For this review, take the finished solid that the model builds, in its own axes (mm). Face numbers are marked on the shaded views. A direction names the side the tool comes from. Round coordinates to 2 decimals unless told otherwise and drop trailing zeros. Order: outer loops, then holes, each group sorted by start corner. A loop starts at its lowest first (then second) coordinate and runs counter-clockwise, first axis right, second up. Notation, with made-up numbers: M 72,3 L 116,3 A15 ccw 116,27 Z; hole C -31.5,67.5 d4. An arc over 180 degrees is marked long. Answer as a JSON object with one key per item and string values.
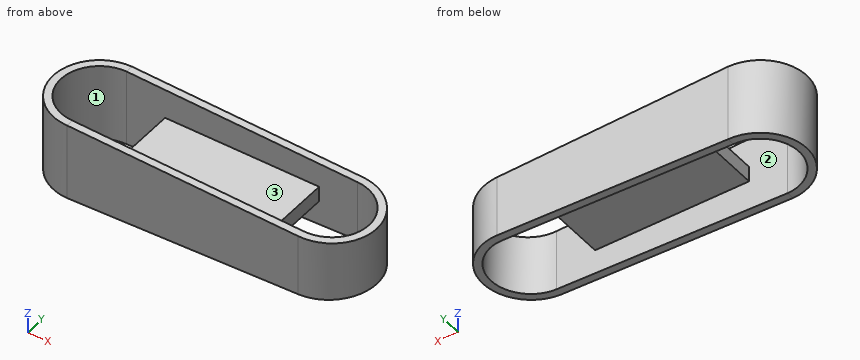
from build123d import *

# Parameters (mm, degrees)
BOSS_EXTRUDE1_DEPTH = 10
SKETCH2_W           = 20
SKETCH2_H           = 2
BOSS_EXTRUDE2_DEPTH = 10
CUT_EXTRUDE1_START  = -12
CUT_EXTRUDE1_DEPTH  = 12


# Read off the part's stored shape, not the designer's step: Cut-Extrude1
with BuildPart() as part:
    # Sketch1 → Boss-Extrude1 (new body)
    with BuildSketch(Plane.XY):
        with BuildLine():
            Line((0, -6), (-30, -6))
            ThreePointArc((-30, -6), (-36, 0), (-30, 6))
            Line((-30, 6), (0, 6))
            ThreePointArc((0, 6), (6, 0), (0, -6))
        make_face()
        with BuildLine():
            Line((-30, 5), (0, 5))
            ThreePointArc((0, 5), (5, 0), (0, -5))
            Line((0, -5), (-30, -5))
            ThreePointArc((-30, -5), (-35, 0), (-30, 5))
        make_face(mode=Mode.SUBTRACT)
    extrude(amount=BOSS_EXTRUDE1_DEPTH)

    # Sketch2 → Boss-Extrude2 (add)
    with BuildSketch(Plane(origin=(0, -5, 0), x_dir=(1, 0, 0), z_dir=(0, 1, 0))):
        with Locations((-15, -5)):
            Rectangle(SKETCH2_W, SKETCH2_H)
    extrude(amount=BOSS_EXTRUDE2_DEPTH)

    # Cut-Extrude1 outline → Cut-Extrude1 (cut)
    with BuildSketch(Plane(origin=(0, 6, 0), x_dir=(1, 0, 0), z_dir=(0, 1, 0)).offset(CUT_EXTRUDE1_START)):
        Polygon((6, -8.8), (-30, -10), (7, -10), (7, -8.766666667), align=None)
        Polygon((6, -1.2), (7, -1.233333333), (7, 0), (-30, 0), align=None)
    extrude(amount=CUT_EXTRUDE1_DEPTH, mode=Mode.SUBTRACT)


solid = part.part
1) Add section B-B on y = 1.75. State the section outline as (x, z) points.
Geometry check:
{"outline": "M -35.74,0 L -34.68,0 L -34.68,10 L -35.74,10 Z; M -25,4 L -5,4 L -5,6 L -25,6 Z; M 4.68,1.16 L 5.74,1.19 L 5.74,8.81 L 4.68,8.84 Z"}
2) Add section A-A on z = 7. State the section outline as (x, y) points.
Geometry check:
{"outline": "M -30,-6 L 0,-6 A6 ccw 0,6 L -30,6 A6 ccw Z; hole M -30,-5 L 0,-5 A5 ccw 0,5 L -30,5 A5 ccw Z"}
3) Add section C-C on x = -12. State the section outline as (y, z) points.
Geometry check:
{"outline": "M -6,0.6 L -5,0.6 L -5,4 L 5,4 L 5,0.6 L 6,0.6 L 6,9.4 L 5,9.4 L 5,6 L -5,6 L -5,9.4 L -6,9.4 Z"}
4) Machinability: for the marked faces 1, 2 and 3, which of the approach directions +Z, -Z, +X, -X, +Y, -Y give a long, thin tool a straight path to every point of the face, cutting with its end or side? Answer none if there is none.
Geometry check:
{"face 1": "+Z, -Z", "face 2": "none", "face 3": "+Z"}
5) For L1, parallel to Y at x = -22, z = 6.25; L2, parallel to Z at x = -14, y = -4.75; L3, parallel to X at y = -0.25, z = 3.25, list the stretches that pass through material, from the lowest coordinate up.
Geometry check:
{"L1": "y = -6 to -5, 5 to 6", "L2": "z = 4 to 6", "L3": "x = -35.99 to -34.99, 4.99 to 5.99"}
6) Add section D-D on z = 5.25. State the section outline as (x, y) points, and give its area (3 significant figures).
Geometry check:
{"outline": "M -30,-6 L 0,-6 A6 ccw 0,6 L -30,6 A6 ccw Z; hole M -30,-5 L -25,-5 L -25,5 L -30,5 A5 ccw Z; hole M -5,-5 L 0,-5 A5 ccw 0,5 L -5,5 Z", "area": "295 mm²"}
7) Insertion check: P1, Ø4, axis at x = -31.5, y = 1, coming from the +Z side; P2, Ø4, axis at y = 0.5, z = 1.5, coming from the -X side; P3, Ø4, axis at x = -7, y = -0.5, coming from the -Z side; P4, Ø2, axis at y = -2, z = 4.5, coming from the -X side. Each pin has a flat end and moves straight along its axis. Give the tip position at first contact, or say it passes through.
Geometry check:
{"P1": "passes through", "P2": "stops at x = -36", "P3": "stops at z = 4", "P4": "stops at x = -35.92"}
